Geometry check sheet. Reference: the model listing, model coordinates, mm. Face numbers are marked on the shaded views. Round coordinates to 2 decimals unless told otherwise and drop trailing zeros. Order: outer loops, then holes, each group sorted by start corner. A loop starts at its lowest first (then second) coordinate and runs counter-clockwise, first axis right, second up. Notation, with made-up numbers: (16.5, 62) - (51.5, 62) arc R16 ccw to (51.5, 82) - close; hole circle Ø1 at (21.25, 83.25). An arc over 180 degrees is marked (long way). Use a Markdown table: item, result. Add a question column.
(1) Thickness scan on line 1 along X through (y, z) = (-7.25, 9); line 2 along X through (y, z) = (-7, 6.5); line 3 along Z through (x, y) = (48, -7). Record the ranges inside material, lowest first. Write a range as [from, to].
(2) Gauge pin test, flat ends, axial feed: P1, Ø1.5, axis at x = -24.5, z = 62, coming from the +Y side; P2, Ø2, axis at y = -6, z = 93, coming from the -X side; P3, Ø3, axis at y = -2.5, z = 61, coming from the -X side; P4, Ø3, axis at x = -37, y = -6, coming from the +Z side. Record the tip position at first contact, or that the pin passes through.
(3) Section check B-B on y = -6.25. Record the boundary of the cut face in (x, z).
(4) Section check A-A on x = 48. Record the boundary of the cut face in (y, z), then the cut area to 3 significant figures.
(5) Mould release check, pull along X, two halves, no side actions. Record for the marked faces 1, 2 and 3: released by +X, released by -X, zero draft, split by the parting line, or undercut.
(6) Section check D-D on x = 8. Record the boundary of the cut face in (y, z), then the cut area to 3 significant figures.
(7) Section check C-C on z = 7. Record the boundary of the cut face in (x, y), then the cut area to 3 significant figures.
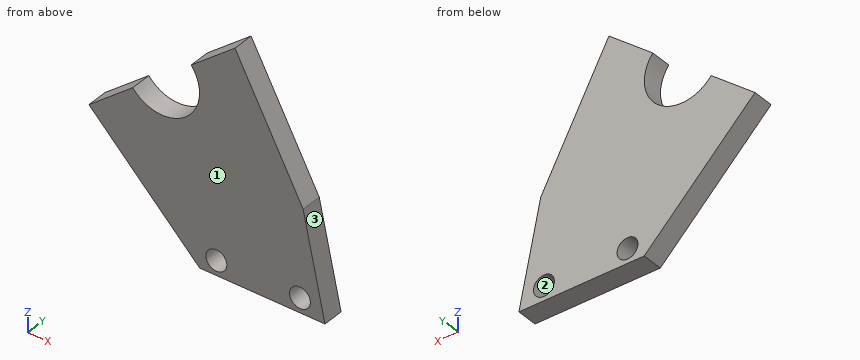
Solid Edge part; units mm, degrees
sketch "Sketch1" plane through (0, 0, 0) normal (0, -1, 0) x (1, 0, 0)
  line L0 (-53.033, 53.033) -> (0, 0)
  line L1 (0, 0) -> (60, 0)
  line L2 (60, 0) -> (49.5321, 48.892)
  line L3 (49.5321, 48.892) -> (16.898, 109.6868)
  line L4 (-53.033, 53.033) -> (16.898, 109.6868)
  dimension "D1" = 53.033
  dimension "D2" = 60
  dimension "D3" = 49.5321
  dimension "D4" = 53.033
extrude "Protrusion1" add sketch "Sketch1" along normal blind 10
sketch "Sketch2" plane through (-1.5165, 0, 51.9599) normal (0, 1, 0) x (-1, 0, 0)
  line L0 (2.5648, 40.7308) -> (30.5372, 18.0693)
  arc A0 (30.5372, 18.0693) -> (2.5648, 40.7308) centre (16.551, 29.4) cw
  dimension "D1" = 2.5648
extrude "Cutout1" cut sketch "Sketch2" against normal up to next
sketch "Sketch3" plane through (3.4835, 0, 54.8434) normal (0, 1, 0) x (-1, 0, 0)
  circle A0 centre (-44.5165, -47.8434) radius 5
  circle A1 centre (-4.5165, -47.8434) radius 5
  dimension "D1" = 44.5165
extrude "Cutout2" cut sketch "Sketch3" against normal up to next
Check sheet entries:
| question | item | result |
|---|---|---|
| 1 | line 1 | x = [-9, 3.42], [12.58, 43.42], [52.58, 58.07] |
| 1 | line 2 | x = [-6.5, 3.03], [12.97, 43.03], [52.97, 58.61] |
| 1 | line 3 | z = [0, 2], [12, 51.75] |
| 2 | P1 | stops at y = 0 |
| 2 | P2 | stops at x = -4.08 |
| 2 | P3 | stops at x = -45.05 |
| 2 | P4 | stops at z = 67.24 |
| 3 | outline | (-53.03, 53.03) - (0, 0) - (60, 0) - (49.53, 48.89) - (16.9, 109.69) - (-4.08, 92.69) arc R18 cw to (-32.05, 70.03) - close; hole circle Ø10 at (8, 7); hole circle Ø10 at (48, 7) |
| 4 | outline | (-10, 0) - (0, 0) - (0, 2) - (-10, 2) - close; (-10, 12) - (0, 12) - (0, 51.75) - (-10, 51.75) - close |
| 4 | area | 417 mm2 |
| 5 | face 1 | zero draft |
| 5 | face 2 | undercut |
| 5 | face 3 | released by +X |
| 6 | outline | (-10, 0) - (0, 0) - (0, 2) - (-10, 2) - close; (-10, 12) - (0, 12) - (0, 102.48) - (-10, 102.48) - close |
| 6 | area | 925 mm2 |
| 7 | outline | (-7, -10) - (3, -10) - (3, 0) - (-7, 0) - close; (13, -10) - (43, -10) - (43, 0) - (13, 0) - close; (53, -10) - (58.5, -10) - (58.5, 0) - (53, 0) - close |
| 7 | area | 455 mm2 |
